```python
from build123d import *

# Parameters (mm, degrees)
SKETCH15_W           = 78
SKETCH15_H           = 55
BOSS_EXTRUDE9_DEPTH  = 50
SKETCH16_W           = 58
SKETCH16_H           = 32
CUT_EXTRUDE3_DEPTH   = 50
SKETCH17_R           = 20
BOSS_EXTRUDE10_DEPTH = 20
BOSS_EXTRUDE11_DEPTH = 15


with BuildPart() as part:
    # Sketch15 → Boss-Extrude9 (new body)
    with BuildSketch(Plane.XY):
        with Locations((39, 27.5)):
            Rectangle(SKETCH15_W, SKETCH15_H)
    extrude(amount=BOSS_EXTRUDE9_DEPTH)

    # Sketch16 → Cut-Extrude3 (cut)
    with BuildSketch(Plane.XY.offset(50)):
        with Locations((39, 16)):
            Rectangle(SKETCH16_W, SKETCH16_H)
    extrude(amount=-CUT_EXTRUDE3_DEPTH, mode=Mode.SUBTRACT)

    # Sketch17 → Boss-Extrude10 (add)
    with BuildSketch(Plane(origin=(0, 0, 0), x_dir=(-1, 0, 0), z_dir=(0, 0, -1))):
        with Locations((-39, 55)):
            Circle(SKETCH17_R)
    extrude(amount=-BOSS_EXTRUDE10_DEPTH)

    # Sketch21 → Boss-Extrude11 (add, symmetric)
    with BuildSketch(Plane(origin=(0, 0, 25), x_dir=(-1, 0, 0), z_dir=(0, 0, -1))):
        Polygon((-9.5, 0), (18, 0), (18, 20), (3.5, 65), (-9.5, 65), align=None)
    boss_extrude11 = extrude(amount=BOSS_EXTRUDE11_DEPTH, both=True)

    # Mirror4: Boss-Extrude11 across plane
    add(boss_extrude11.mirror(Plane.ZY.offset(-39)))


solid = part.part
```
Here's how the part is built. I have some questions about the finished solid (model axes, mm). A direction names the side the tool comes from. Round coordinates to 2 decimals unless told otherwise and drop trailing zeros. Order: outer loops, then holes, each group sorted by start corner. A loop starts at its lowest first (then second) coordinate and runs counter-clockwise, first axis right, second up. Notation, with made-up numbers: (27, 50) -> (69, 50) arc R29 cw to (69, 82) -> close; hole circle Ø11 at (70.25, -34). An arc over 180 degrees is marked (long way). Use a Markdown table: item, result. Add a question column.
(1) For pin 1 Ø5 at (y, z) = (36, 46.5) entering from +X; pin 2 Ø8 at (x, y) = (-7.5, 40.5) entering from -Z; pin 3 Ø3 at (y, z) = (19.5, 45.5) entering from -X, each with a flat end and sliding along its axis, tell me the tip position at first contact or that it passes through.
(2) Suppose I cut it at A-A, the plane z = 17.5. Please give me the cut outline in (x, y), and give its area (3 significant figures).
(3) Suppose I cut it at C-C, the plane y = 63. Please give me the cut outline in (x, z), and give its area (3 significant figures).
(4) Suppose I cut it at D-D, the plane z = 23.5. Please give me the cut outline in (x, y), and give its area (3 significant figures).
(5) I need wall thicknesses on line 1 along X through (y, z) = (10, 31); line 2 along X through (y, z) = (12, 7.5); line 3 along X through (y, z) = (41, 4.5). Which ranges of each line are inside material? Lowest first, please.
(6) Suppose I cut it at B-B, the plane x = 4. Please give me the cut outline in (y, z).
(7) For faces 5 (the face through (0, 27, 5)), 6 (the face through (75, 65, 25)), 7 (the face through (78, 27, 5)), 8 (the face through (39, 63, 20)), which set-ups out of +Z, -Z, +X, -X, +Y, -Y let a thin tool reach every point of the face, with its end or its side?
(8) If we mould it in two halves opening along X, with no side actions, what happens to faces 1 (the face through (68, 16, 25)), 2 (the face through (38, 55, 30)), 3 (the face through (-18, 10, 25)), 4 (the face through (-1, 0, 25))? For each: released by +X, released by -X, zero draft, split by the parting line, or undercut.
Verdict:
| question | item | result |
|---|---|---|
| 1 | pin 1 | x = 78 |
| 1 | pin 2 | z = 10 |
| 1 | pin 3 | x = 0 |
| 2 | outline | (-18, 0) -> (10, 0) -> (10, 32) -> (68, 32) -> (68, 0) -> (96, 0) -> (96, 20) -> (81.5, 65) -> (68.5, 65) -> (68.5, 55) -> (59, 55) arc R20 ccw to (19, 55) -> (9.5, 55) -> (9.5, 65) -> (-3.5, 65) -> (-18, 20) -> close |
| 2 | area | 4,940 mm2 |
| 3 | outline | (-4.14, 10) -> (9.5, 10) -> (9.5, 40) -> (-4.14, 40) -> close; (20.67, 0) -> (57.33, 0) -> (57.33, 20) -> (20.67, 20) -> close; (68.5, 10) -> (82.14, 10) -> (82.14, 40) -> (68.5, 40) -> close |
| 3 | area | 1,550 mm2 |
| 4 | outline | (-18, 0) -> (10, 0) -> (10, 32) -> (68, 32) -> (68, 0) -> (96, 0) -> (96, 20) -> (81.5, 65) -> (68.5, 65) -> (68.5, 55) -> (9.5, 55) -> (9.5, 65) -> (-3.5, 65) -> (-18, 20) -> close |
| 4 | area | 4,310 mm2 |
| 5 | line 1 | -18 to 10, 68 to 96 |
| 5 | line 2 | 0 to 10, 68 to 78 |
| 5 | line 3 | 0 to 78 |
| 6 | outline | (0, 0) -> (55, 0) -> (55, 10) -> (65, 10) -> (65, 40) -> (55, 40) -> (55, 50) -> (0, 50) -> close |
| 7 | face 5 | -Z, -X, +Y, -Y |
| 7 | face 6 | +Z, -Z, +X, +Y |
| 7 | face 7 | -Z, +X, +Y, -Y |
| 7 | face 8 | +Z, +Y |
| 8 | face 1 | undercut |
| 8 | face 2 | undercut |
| 8 | face 3 | released by -X |
| 8 | face 4 | zero draft |
